For this review, take the finished solid that the model builds, in its own axes (mm). A direction names the side the tool comes from. Round coordinates to 2 decimals unless told otherwise and drop trailing zeros. Order: outer loops, then holes, each group sorted by start corner. A loop starts at its lowest first (then second) coordinate and runs counter-clockwise, first axis right, second up. Notation, with made-up numbers: M -13.75,44 L -5.75,44 A15 cw -5.75,48 Z; hole C 34.25,62.25 d4. An arc over 180 degrees is marked long. Answer in a Markdown table with one row per item. Add a question column.
```python
from build123d import *

# Parameters (mm, degrees)
SKETCH2_W                       = 42.3
SKETCH2_H                       = 130
SKETCH2_R                       = 12.5
SKETCH2_R_2                     = 4.1
BOSS_EXTRUDE1_DEPTH             = 6.35
TAP_DRILL_FOR_M3X0_5_TAP1_D     = 2.5
TAP_DRILL_FOR_M3X0_5_TAP1_DEPTH = 21.15
TAP_DRILL_FOR_M3X0_5_TAP1_TIP   = 0.751075774
TAP_DRILL_FOR_M3X0_5_TAP2_D     = 2.5
F_1_4_CLEARANCE_HOLE1_D         = 6.7564
BOSS_EXTRUDE2_DEPTH             = 6.35
TAP_DRILL_FOR_M4X0_7_TAP1_D     = 3.3


with BuildPart() as part:
    # Sketch2 → Boss-Extrude1 (new body)
    with BuildSketch(Plane.XY):
        with Locations((0, 43.85)):
            Rectangle(SKETCH2_W, SKETCH2_H)
        Circle(SKETCH2_R, mode=Mode.SUBTRACT)
        with Locations((0, 25)):
            Circle(SKETCH2_R_2, mode=Mode.SUBTRACT)
        with Locations((0, 50)):
            Circle(SKETCH2_R_2, mode=Mode.SUBTRACT)
    extrude(amount=BOSS_EXTRUDE1_DEPTH)

    # Tap Drill for M3x0.5 Tap1
    with Locations(Plane(origin=(21.15, 0, 0), x_dir=(0, 0, 1), z_dir=(1, 0, 0))):
        with Locations((3.175, -50), (3.175, 0), (3.175, -25)):
            Hole(TAP_DRILL_FOR_M3X0_5_TAP1_D / 2, depth=TAP_DRILL_FOR_M3X0_5_TAP1_DEPTH)
            with Locations((0, 0, -(TAP_DRILL_FOR_M3X0_5_TAP1_DEPTH + TAP_DRILL_FOR_M3X0_5_TAP1_TIP / 2))):  # 118° drill point
                Cone(0, TAP_DRILL_FOR_M3X0_5_TAP1_D / 2, TAP_DRILL_FOR_M3X0_5_TAP1_TIP, mode=Mode.SUBTRACT)

    # Tap Drill for M3x0.5 Tap2 (through all)
    with Locations(Plane.XY.offset(6.35)):
        with Locations((-15.5, 15.5), (-15.5, -15.5), (15.5, -15.5), (15.5, 15.5)):
            Hole(TAP_DRILL_FOR_M3X0_5_TAP2_D / 2)

    # 1/4 Clearance Hole1 (through all)
    with Locations(Plane.XY.offset(6.35)):
        with Locations((-13.15, 86.85), (-13.15, 100.85)):
            Hole(F_1_4_CLEARANCE_HOLE1_D / 2)

    # Sketch13 → Boss-Extrude2 (add)
    with BuildSketch(Plane.XY.offset(6.35)):
        Polygon((-21.15, 8.85), (-51.15, 26.170508076), (-51.15, 76.170508076), (-21.15, 93.491016151), align=None)
    extrude(amount=-BOSS_EXTRUDE2_DEPTH)

    # Tap Drill for M4x0.7 Tap1 (through all)
    with Locations(Plane.XY.offset(6.35)):
        with Locations((-45.15, 59.170508076), (-21.15, 59.170508076), (-21.15, 43.170508076), (-45.15, 43.170508076)):
            Hole(TAP_DRILL_FOR_M4X0_7_TAP1_D / 2)


solid = part.part
```
1. Consider section A-A on x = 15.5. Write out the cut boundary in (y, z) (3 decimals).
2. Consider section C-C on x = 6. Write out the cut boundary in (y, z) (3 decimals), plus the area to 3 significant figures.
3. Clearance check with flat-ended pins moving along their axes: pin 1 Ø3 at (y, z) = (-6, 3.5) entering from -X; pin 2 Ø2 at (x, y) = (-45.15, 43.17) entering from +Z; pin 3 Ø2 at (y, z) = (25, 3.175) entering from +X. State where each tip first meets the part, or that it passes through.
4. To check wall thickness, follow probe 1 along Y at (x, z) = (0, 5); probe 2 along Z at (x, y) = (17.5, 50) (3 decimals); probe 3 along Y at (x, z) = (-13.15, 1.5). State the ranges of each line that lie inside material, in increasing order. Write a range as [from, to].
5. Consider section D-D on y = 100.85. Write out the cut boundary in (x, z).
6. For faces 4 (the cylindrical face through (12.41, 26.22, 3.45)), 5 (the cylindrical face through (16.421, 16.345, 3.131)), list the 3-axis set-ups (+Z, -Z, +X, -X, +Y, -Y) from which the entire face can be reached by the end or side of a thin tool; tool diameter is ignored.
7. Consider section B-B on y = -15.5. Write out the cut boundary in (x, z).
8. The part is to be moulded in two halves that separate along Y. For faces 1 (the flat face through (-36.36, 84.71, 3.22)), 2 (the cylindrical face through (11.923, 3.755, 3.131)), 3 (the flat face through (0, -21.15, 3)), say which applies: pulls with the +Y half, pulls with the -Y half, needs draft (parallel to the pull), parting line crosses it, or undercut.
Solved:
| question | item | result |
|---|---|---|
| 1 | outline | M -21.15,0 L -16.75,0 L -16.75,6.35 L -21.15,6.35 Z; M -14.25,0 L 14.25,0 L 14.25,6.35 L -14.25,6.35 Z; M 16.75,0 L 108.85,0 L 108.85,6.35 L 16.75,6.35 Z; hole C 0,3.175 d2.5; hole C 25,3.175 d2.5; hole C 50,3.175 d2.5 |
| 2 | outline | M -21.15,0 L -10.966,0 L -10.966,6.35 L -21.15,6.35 Z; M 10.966,0 L 108.85,0 L 108.85,6.35 L 10.966,6.35 Z; hole C 25,3.175 d2.5; hole C 50,3.175 d2.5 |
| 2 | area | 676 mm^2 |
| 3 | pin 1 | stops at x = -21.15 |
| 3 | pin 2 | passes through |
| 3 | pin 3 | stops at x = -3.98 |
| 4 | probe 1 | y = [-21.15, -12.5], [12.5, 20.9], [29.1, 45.9], [54.1, 108.85] |
| 4 | probe 2 | z = [0, 1.925], [4.425, 6.35] |
| 4 | probe 3 | y = [-21.15, 83.47], [90.23, 97.47], [104.23, 108.85] |
| 5 | outline | M -21.15,0 L -16.53,0 L -16.53,6.35 L -21.15,6.35 Z; M -9.77,0 L 21.15,0 L 21.15,6.35 L -9.77,6.35 Z |
| 6 | face 4 | +X |
| 6 | face 5 | +Z, -Z |
| 7 | outline | M -21.15,0 L -16.75,0 L -16.75,6.35 L -21.15,6.35 Z; M -14.25,0 L 14.25,0 L 14.25,6.35 L -14.25,6.35 Z; M 16.75,0 L 21.15,0 L 21.15,6.35 L 16.75,6.35 Z |
| 8 | face 1 | pulls with the +Y half |
| 8 | face 2 | undercut |
| 8 | face 3 | pulls with the -Y half |
